from build123d import *

# Parameters (mm, degrees)
EXTRUDE_246_DEPTH       = 6
CHAMFER_C3_SIZE         = 3
CUT_EXTRUDE_9_1P5_DEPTH = 1.5
CUT_EXTRUDE_1P5_DEPTH   = 1.5
CUT_EXTRUDE_START       = 2.8
SKETCH_4_R              = 3.1
CUT_EXTRUDE_2P8_DEPTH   = 3.2


with BuildPart() as part:
    # 草图1 → Extrude 246 (new body)
    with BuildSketch(Plane.XY):
        Polygon((-31, -60), (31, -60), (36, -50), (38, -45), (38, 50), (28, 66), (-28, 66), (-38, 50), (-38, -45), (-36, -50), align=None)
    extrude(amount=EXTRUDE_246_DEPTH)

    # 橡胶垫全周向心倒角_C3
    # the kernel refuses this chamfer: 3 mm, written as the material it takes off along each edge
    with BuildSketch(Plane(origin=(-40.865297253, -37.836756868, 0), x_dir=(-0.025529280528386825, -0.01021171221135473, 0.9996219169112968), z_dir=(0.3713906763541037, -0.9284766908852594, 0)), Plane(origin=(33.134702747, -57.163243132, 0), x_dir=(0.025529280528386825, -0.01021171221135473, 0.9996219169112968), z_dir=(0.3713906763541037, 0.9284766908852594, 0))) as chamfer_c3_piece_1:
        Polygon((CHAMFER_C3_SIZE * 0.999621916911, -CHAMFER_C3_SIZE * 0.0274958766106), (-CHAMFER_C3_SIZE * 0.0274958766106, -CHAMFER_C3_SIZE * 0.999621916911), (0, 0), align=None)
    extrude(amount=20.815262735, mode=Mode.SUBTRACT)
    with BuildSketch(Plane(origin=(-38, 57.715048964, 0), x_dir=(-0.027495876610586778, 0, 0.9996219169112968), z_dir=(0, -1, 0)), Plane(origin=(38, -52.715048964, 0), x_dir=(0.027495876610586778, 0, 0.9996219169112968), z_dir=(0, 1, 0))) as chamfer_c3_piece_2:
        Polygon((CHAMFER_C3_SIZE * 0.999621916911, -CHAMFER_C3_SIZE * 0.0274958766106), (-CHAMFER_C3_SIZE * 0.0274958766106, -CHAMFER_C3_SIZE * 0.999621916911), (0, 0), align=None)
    extrude(amount=110.430097928, mode=Mode.SUBTRACT)
    with BuildSketch(Plane(origin=(-23.911032227, 72.542348437, 0), x_dir=(-0.023316456732911096, 0.014572785458069436, 0.9996219169112968), z_dir=(-0.52999894000318, -0.847998304005088, 0)), Plane(origin=(42.088967773, 43.457651563, 0), x_dir=(0.02331645673290944, 0.014572785458068402, 0.9996219169112968), z_dir=(-0.52999894000318, 0.847998304005088, 0))) as chamfer_c3_piece_3:
        Polygon((CHAMFER_C3_SIZE * 0.999621916911, -CHAMFER_C3_SIZE * 0.0274958766106), (-CHAMFER_C3_SIZE * 0.0274958766106, -CHAMFER_C3_SIZE * 0.999621916911), (0, 0), align=None)
    extrude(amount=34.298060192, mode=Mode.SUBTRACT)
    with BuildSketch(Plane(origin=(35.715048964, 66, 0), x_dir=(0, 0.027495876610586778, 0.9996219169112968), z_dir=(-1, 0, 0))) as chamfer_c3_piece_4:
        Polygon((CHAMFER_C3_SIZE * 0.999621916911, -CHAMFER_C3_SIZE * 0.0274958766106), (-CHAMFER_C3_SIZE * 0.0274958766106, -CHAMFER_C3_SIZE * 0.999621916911), (0, 0), align=None)
    extrude(amount=71.430097928, mode=Mode.SUBTRACT)
    with BuildSketch(Plane(origin=(27.549725213, -66.900549573, 0), x_dir=(0.024593059680886438, -0.012296529840443219, 0.9996219169112968), z_dir=(0.447213595499958, 0.894427190999916, 0)), Plane(origin=(-39.450274787, -43.099450427, 0), x_dir=(-0.024593059680884596, -0.012296529840442298, 0.9996219169112968), z_dir=(0.447213595499958, -0.894427190999916, 0))) as chamfer_c3_piece_5:
        Polygon((CHAMFER_C3_SIZE * 0.999621916911, -CHAMFER_C3_SIZE * 0.0274958766106), (-CHAMFER_C3_SIZE * 0.0274958766106, -CHAMFER_C3_SIZE * 0.999621916911), (0, 0), align=None)
    extrude(amount=26.610437815, mode=Mode.SUBTRACT)
    with BuildSketch(Plane(origin=(-38.715048964, -60, 0), x_dir=(0, -0.027495876610586778, 0.9996219169112968), z_dir=(1, 0, 0))) as chamfer_c3_piece_6:
        Polygon((CHAMFER_C3_SIZE * 0.999621916911, -CHAMFER_C3_SIZE * 0.0274958766106), (-CHAMFER_C3_SIZE * 0.0274958766106, -CHAMFER_C3_SIZE * 0.999621916911), (0, 0), align=None)
    extrude(amount=77.430097928, mode=Mode.SUBTRACT)

    # 草图2 → 鞋底横向等距防滑槽_节距9_深1p5 (cut)
    with BuildSketch(Plane.XY):
        with BuildLine():
            Line((-28.9, -46.1), (28.9, -46.1))
            ThreePointArc((28.9, -46.1), (30, -45), (28.9, -43.9))
            Line((28.9, -43.9), (-28.9, -43.9))
            ThreePointArc((-28.9, -43.9), (-30, -45), (-28.9, -46.1))
        make_face()
        with BuildLine():
            Line((-28.9, -37.1), (28.9, -37.1))
            ThreePointArc((28.9, -37.1), (30, -36), (28.9, -34.9))
            Line((28.9, -34.9), (-28.9, -34.9))
            ThreePointArc((-28.9, -34.9), (-30, -36), (-28.9, -37.1))
        make_face()
        with BuildLine():
            Line((-28.9, -28.1), (28.9, -28.1))
            ThreePointArc((28.9, -28.1), (30, -27), (28.9, -25.9))
            Line((28.9, -25.9), (-28.9, -25.9))
            ThreePointArc((-28.9, -25.9), (-30, -27), (-28.9, -28.1))
        make_face()
        with BuildLine():
            Line((-28.9, -19.1), (28.9, -19.1))
            ThreePointArc((28.9, -19.1), (30, -18), (28.9, -16.9))
            Line((28.9, -16.9), (-28.9, -16.9))
            ThreePointArc((-28.9, -16.9), (-30, -18), (-28.9, -19.1))
        make_face()
        with BuildLine():
            Line((-28.9, -10.1), (28.9, -10.1))
            ThreePointArc((28.9, -10.1), (30, -9), (28.9, -7.9))
            Line((28.9, -7.9), (-28.9, -7.9))
            ThreePointArc((-28.9, -7.9), (-30, -9), (-28.9, -10.1))
        make_face()
        with BuildLine():
            Line((-28.9, -1.1), (28.9, -1.1))
            ThreePointArc((28.9, -1.1), (30, 0), (28.9, 1.1))
            Line((28.9, 1.1), (-28.9, 1.1))
            ThreePointArc((-28.9, 1.1), (-30, 0), (-28.9, -1.1))
        make_face()
        with BuildLine():
            Line((-28.9, 7.9), (28.9, 7.9))
            ThreePointArc((28.9, 7.9), (30, 9), (28.9, 10.1))
            Line((28.9, 10.1), (-28.9, 10.1))
            ThreePointArc((-28.9, 10.1), (-30, 9), (-28.9, 7.9))
        make_face()
        with BuildLine():
            Line((-28.9, 16.9), (28.9, 16.9))
            ThreePointArc((28.9, 16.9), (30, 18), (28.9, 19.1))
            Line((28.9, 19.1), (-28.9, 19.1))
            ThreePointArc((-28.9, 19.1), (-30, 18), (-28.9, 16.9))
        make_face()
        with BuildLine():
            Line((-28.9, 25.9), (28.9, 25.9))
            ThreePointArc((28.9, 25.9), (30, 27), (28.9, 28.1))
            Line((28.9, 28.1), (-28.9, 28.1))
            ThreePointArc((-28.9, 28.1), (-30, 27), (-28.9, 25.9))
        make_face()
        with BuildLine():
            Line((-28.9, 34.9), (28.9, 34.9))
            ThreePointArc((28.9, 34.9), (30, 36), (28.9, 37.1))
            Line((28.9, 37.1), (-28.9, 37.1))
            ThreePointArc((-28.9, 37.1), (-30, 36), (-28.9, 34.9))
        make_face()
        with BuildLine():
            Line((-28.9, 43.9), (28.9, 43.9))
            ThreePointArc((28.9, 43.9), (30, 45), (28.9, 46.1))
            Line((28.9, 46.1), (-28.9, 46.1))
            ThreePointArc((-28.9, 46.1), (-30, 45), (-28.9, 43.9))
        make_face()
        with BuildLine():
            Line((-28.9, 52.9), (28.9, 52.9))
            ThreePointArc((28.9, 52.9), (30, 54), (28.9, 55.1))
            Line((28.9, 55.1), (-28.9, 55.1))
            ThreePointArc((-28.9, 55.1), (-30, 54), (-28.9, 52.9))
        make_face()
    extrude(amount=CUT_EXTRUDE_9_1P5_DEPTH, mode=Mode.SUBTRACT)

    # 草图3 → 鞋底纵向分区槽_深1p5 (cut)
    with BuildSketch(Plane.XY):
        with BuildLine():
            Line((-14.1, -46), (-13.9, -46))
            ThreePointArc((-13.9, -46), (-13.192893219, -45.707106781), (-12.9, -45))
            Line((-12.9, -45), (-12.9, 51))
            ThreePointArc((-12.9, 51), (-13.192893219, 51.707106781), (-13.9, 52))
            Line((-13.9, 52), (-14.1, 52))
            ThreePointArc((-14.1, 52), (-14.807106781, 51.707106781), (-15.1, 51))
            Line((-15.1, 51), (-15.1, -45))
            ThreePointArc((-15.1, -45), (-14.807106781, -45.707106781), (-14.1, -46))
        make_face()
        with BuildLine():
            Line((13.9, -46), (14.1, -46))
            ThreePointArc((14.1, -46), (14.807106781, -45.707106781), (15.1, -45))
            Line((15.1, -45), (15.1, 51))
            ThreePointArc((15.1, 51), (14.807106781, 51.707106781), (14.1, 52))
            Line((14.1, 52), (13.9, 52))
            ThreePointArc((13.9, 52), (13.192893219, 51.707106781), (12.9, 51))
            Line((12.9, 51), (12.9, -45))
            ThreePointArc((12.9, -45), (13.192893219, -45.707106781), (13.9, -46))
        make_face()
    extrude(amount=CUT_EXTRUDE_1P5_DEPTH, mode=Mode.SUBTRACT)

    # 草图4 → 底部螺钉头背面避让_保留2p8底厚 (cut)
    with BuildSketch(Plane.XY.offset(CUT_EXTRUDE_START)):
        with Locations((-22, -56)):
            Circle(SKETCH_4_R)
        with Locations((-25, 53)):
            Circle(SKETCH_4_R)
        with Locations((-34, -43)):
            Circle(SKETCH_4_R)
        with Locations((-34, 43)):
            Circle(SKETCH_4_R)
        with Locations((22, -56)):
            Circle(SKETCH_4_R)
        with Locations((25, 53)):
            Circle(SKETCH_4_R)
        with Locations((34, -43)):
            Circle(SKETCH_4_R)
        with Locations((34, 43)):
            Circle(SKETCH_4_R)
    extrude(amount=CUT_EXTRUDE_2P8_DEPTH, mode=Mode.SUBTRACT)


solid = part.part
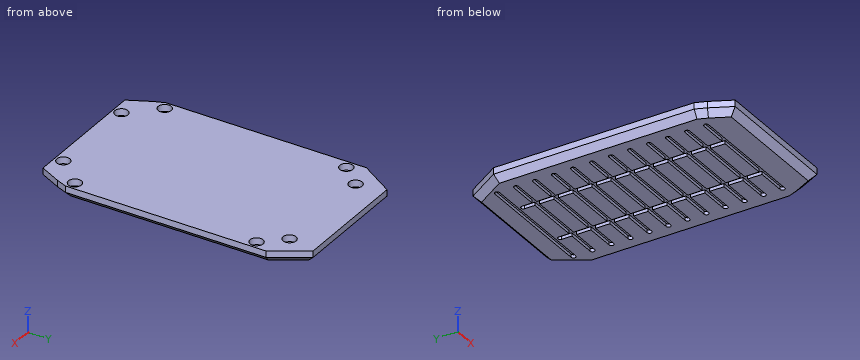
Model file for the job. Use its own axes, mm. Give positions to 0.01 mm unless a question says otherwise; leave off trailing zeros. Loops run counter-clockwise (first coordinate to the right, second up) from the corner with the lowest first, then second, coordinate; pieces in that order, holes last. Notation, with made-up numbers: (35, 22) -> (77, 22) arc R17 cw to (77, 55) -> close; hole circle Ø6 at (38, 24.25). An arc over 180 degrees is marked (long way). Use a Markdown table: item, result. Add a question column.
(1) Slice it at A-A on y = 15.5. List the corners of the cut face in (x, z).
(2) Wall check: line 1 along Y through (x, z) = (34, 5.5); line 2 along Z through (x, y) = (-4.5, -17); line 3 along Y through (x, z) = (-25.5, 4.5). Give the ranges that are in metal, low to high.
(3) Drop flat-ended pins along their axis: pin 1 Ø5 at (x, y) = (34, -43) entering from +Z; pin 2 Ø0.8 at (x, z) = (25, 1) entering from +Y; pin 3 Ø1.6 at (x, z) = (22, 1) entering from +Y. Give the stop position or say it passes through.
Filled sheet:
| question | item | result |
|---|---|---|
| 1 | outline | (-38, 3) -> (-35, 0) -> (-15.1, 0) -> (-15.1, 1.5) -> (-12.9, 1.5) -> (-12.9, 0) -> (12.9, 0) -> (12.9, 1.5) -> (15.1, 1.5) -> (15.1, 0) -> (35, 0) -> (38, 3) -> (38, 6) -> (-38, 6) -> close |
| 2 | line 1 | -54 to -46.1, -39.9 to 39.9, 46.1 to 56.4 |
| 2 | line 2 | 1.5 to 6 |
| 2 | line 3 | -60 to 49.94, 56.06 to 66 |
| 3 | pin 1 | z = 2.8 |
| 3 | pin 2 | y = 64.4 |
| 3 | pin 3 | y = 64.8 |
